from build123d import *

# Parameters (mm, degrees)
SKETCH1_R           = 12.7
SKETCH1_R_2         = 1.65
BOSS_EXTRUDE1_DEPTH = 12.7
SKETCH2_R           = 1.65
CUT_EXTRUDE1_DEPTH  = 12.7
SKETCH3_R           = 2.77495
CUT_EXTRUDE3_DEPTH  = 1.99898
SKETCH7_R           = 1.65
BOSS_EXTRUDE2_DEPTH = 10.70102
SKETCH8_R           = 1.65
BOSS_EXTRUDE3_DEPTH = 10.70102
SKETCH9_R           = 1.65
BOSS_EXTRUDE4_DEPTH = 10.70102
SKETCH10_R          = 1.65
BOSS_EXTRUDE5_DEPTH = 10.70102
SKETCH12_R          = 1.25
CUT_EXTRUDE4_DEPTH  = 12.7
SKETCH11_R          = 1.25
CUT_EXTRUDE5_DEPTH  = 12.7


with BuildPart() as part:
    # Sketch1 → Boss-Extrude1 (new body)
    with BuildSketch(Plane(origin=(0, 0, 0), x_dir=(1, 0, 0), z_dir=(0, 1, 0))):
        with BuildLine():
            Line((21.686311219, 59.206008809), (23.227161891, 57.665158137))
            ThreePointArc((23.227161891, 57.665158137), (23.323849078, 57.508955756), (23.357596674, 57.328376976))
            Line((23.357596674, 57.328376976), (23.357596674, 26.344510207))
            ThreePointArc((23.357596674, 26.344510207), (23.323849078, 26.163931427), (23.227161891, 26.007729046))
            Line((23.227161891, 26.007729046), (21.686311219, 24.466878374))
            ThreePointArc((21.686311219, 24.466878374), (21.530108838, 24.370191187), (21.349530059, 24.336443591))
            Line((21.349530059, 24.336443591), (-9.634336711, 24.336443591))
            ThreePointArc((-9.634336711, 24.336443591), (-9.814915491, 24.370191187), (-9.971117871, 24.466878374))
            Line((-9.971117871, 24.466878374), (-11.511968543, 26.007729046))
            ThreePointArc((-11.511968543, 26.007729046), (-11.60865573, 26.163931427), (-11.642403326, 26.344510207))
            Line((-11.642403326, 26.344510207), (-11.642403326, 57.328376976))
            ThreePointArc((-11.642403326, 57.328376976), (-11.60865573, 57.508955756), (-11.511968543, 57.665158137))
            Line((-11.511968543, 57.665158137), (-9.971117871, 59.206008809))
            ThreePointArc((-9.971117871, 59.206008809), (-9.814915491, 59.302695995), (-9.634336711, 59.336443591))
            Line((-9.634336711, 59.336443591), (21.349530059, 59.336443591))
            ThreePointArc((21.349530059, 59.336443591), (21.530108838, 59.302695995), (21.686311219, 59.206008809))
        make_face()
        with Locations(Location((5.857596674, 41.836443591, 0), (0, 0, 90))):
            Circle(SKETCH1_R, mode=Mode.SUBTRACT)
        with Locations(Location((18.857596674, 54.836443591, 0), (0, 0, 90))):
            Circle(SKETCH1_R_2, mode=Mode.SUBTRACT)
        with Locations(Location((18.857596674, 28.836443591, 0), (0, 0, 90))):
            Circle(SKETCH1_R_2, mode=Mode.SUBTRACT)
        with Locations(Location((-7.142403326, 54.836443591, 0), (0, 0, 90))):
            Circle(SKETCH1_R_2, mode=Mode.SUBTRACT)
        with Locations(Location((-7.142403326, 28.836443591, 0), (0, 0, 90))):
            Circle(SKETCH1_R_2, mode=Mode.SUBTRACT)
    extrude(amount=BOSS_EXTRUDE1_DEPTH)

    # Sketch2 → Cut-Extrude1 (cut)
    with BuildSketch(Plane.XY.offset(-24.336443591)):
        with Locations((-1.888370018, 6.35)):
            Circle(SKETCH2_R)
        with Locations((13.603563366, 6.35)):
            Circle(SKETCH2_R)
        with Locations((5.857596674, 6.35)):
            Circle(SKETCH2_R)
    extrude(amount=-CUT_EXTRUDE1_DEPTH, mode=Mode.SUBTRACT)

    # Sketch3 → Cut-Extrude3 (cut)
    with BuildSketch(Plane(origin=(0, 12.7, 0), x_dir=(1, 0, 0), z_dir=(0, 1, 0))):
        with Locations(Location((-7.142403326, 54.836443591, 0), (0, 0, 270))):
            Circle(SKETCH3_R)
        with Locations(Location((18.857596674, 54.836443591, 0), (0, 0, 270))):
            Circle(SKETCH3_R)
        with Locations(Location((-7.142403326, 28.836443591, 0), (0, 0, 270))):
            Circle(SKETCH3_R)
        with Locations(Location((18.857596674, 28.836443591, 0), (0, 0, 270))):
            Circle(SKETCH3_R)
    extrude(amount=-CUT_EXTRUDE3_DEPTH, mode=Mode.SUBTRACT)

    # Sketch7 → Boss-Extrude2 (add, through all)
    with BuildSketch(Plane(origin=(0, 10.70102, 0), x_dir=(1, 0, 0), z_dir=(0, 1, 0))):
        with Locations((-7.142403326, 28.836443591)):
            Circle(SKETCH7_R)
    extrude(amount=-BOSS_EXTRUDE2_DEPTH)

    # Sketch8 → Boss-Extrude3 (add, through all)
    with BuildSketch(Plane(origin=(0, 10.70102, 0), x_dir=(1, 0, 0), z_dir=(0, 1, 0))):
        with Locations((-7.142403326, 54.836443591)):
            Circle(SKETCH8_R)
    extrude(amount=-BOSS_EXTRUDE3_DEPTH)

    # Sketch9 → Boss-Extrude4 (add, through all)
    with BuildSketch(Plane(origin=(0, 10.70102, 0), x_dir=(1, 0, 0), z_dir=(0, 1, 0))):
        with Locations((18.857596674, 54.836443591)):
            Circle(SKETCH9_R)
    extrude(amount=-BOSS_EXTRUDE4_DEPTH)

    # Sketch10 → Boss-Extrude5 (add, through all)
    with BuildSketch(Plane(origin=(0, 10.70102, 0), x_dir=(1, 0, 0), z_dir=(0, 1, 0))):
        with Locations((18.857596674, 28.836443591)):
            Circle(SKETCH10_R)
    extrude(amount=-BOSS_EXTRUDE5_DEPTH)

    # Sketch12 → Cut-Extrude4 (cut)
    with BuildSketch(Plane(origin=(0, 10.70102, 0), x_dir=(1, 0, 0), z_dir=(0, 1, 0))):
        with Locations(Location((18.857596674, 54.836443591, 0), (0, 0, 270))):
            Circle(SKETCH12_R)
        with Locations(Location((-7.142403326, 28.836443591, 0), (0, 0, 270))):
            Circle(SKETCH12_R)
        with Locations(Location((18.857596674, 28.836443591, 0), (0, 0, 270))):
            Circle(SKETCH12_R)
    extrude(amount=-CUT_EXTRUDE4_DEPTH, mode=Mode.SUBTRACT)

    # Sketch11 → Cut-Extrude5 (cut)
    with BuildSketch(Plane(origin=(0, 10.70102, 0), x_dir=(1, 0, 0), z_dir=(0, 1, 0))):
        with Locations(Location((-7.142403326, 54.836443591, 0), (0, 0, 270))):
            Circle(SKETCH11_R)
    extrude(amount=-CUT_EXTRUDE5_DEPTH, mode=Mode.SUBTRACT)


solid = part.part
Read the model definition and answer for the solid it produces. Units are mm, in the model's axes. A direction names the side the tool comes from. Coordinates: 2 decimals unless noted, no trailing zeros. Loops run counter-clockwise (first coordinate to the right, second up) from the corner with the lowest first, then second, coordinate; pieces in that order, holes last.
Q1. The mould has two halves that part along X. Classify faces 1 (the face through (22.446, 6.261, -58.446)), 2 (the face through (-3.537, 6.423, -27.757)), 3 (the face through (-11.642, 6, -42)): +X half, -X half, draft (parallel to the pull), parting line (faces both ways), or undercut.
Q2. The part is cut by section C-C on z = -49.5. Write down the section's boundary in (x, y).
Q3. Which of the six approach directions +Z, -Z, +X, -X, +Y, -Y give full straight-line access (tool end or side, diameter ignored) to faces 4 (the face through (2.04, 6.26, -53.95)), 5 (the face through (20, 10.701, -54)), 6 (the face through (4.548, 5.346, -26.756))?
Q4. Consider probe 1 along X at (y, z) = (11.5, -29); probe 2 along Z at (x, y) = (19.5, 4); probe 3 along Z at (x, y) = (15, 5). Determine where each line is inside the solid, lowest interval first.
Q5. The part is cut by section A-A on y = 6.35. Give the number of separate pieces and of enclosed holes in the cut face, and give its area (3 significant figures).
Q6. Each of these flat-tipped pins is pushed along its axis until it touches: pin 1 Ø3 at (x, z) = (-7.14, -28.84) entering from -Y; pin 2 Ø3 at (x, z) = (18.86, -28.84) entering from +Y. Where does it stop, or does it pass through?
Q7. The part is cut by section B-B on x = 7. Write down the section's boundary in (y, z).
Q8. The part is cut by section D-D on y = 4. Write down the section's boundary in (x, z).
Results below:
1. face 1: +X half
1. face 2: undercut
1. face 3: -X half
2. outline: (-11.64, 0) - (-4.27, 0) - (-4.27, 12.7) - (-11.64, 12.7) - close; (15.98, 0) - (23.36, 0) - (23.36, 12.7) - (15.98, 12.7) - close
3. face 4: +Y, -Y
3. face 5: +Y
3. face 6: +Z
4. probe 1: x = -11.64 to -9.91, -4.37 to 16.09, 21.63 to 23.36
4. probe 2: z = -59.34 to -55.91, -53.76 to -29.91, -27.76 to -24.34
4. probe 3: z = -59.34 to -50.65, -33.02 to -24.34
5. separate pieces: 3
5. enclosed holes: 4
5. area: 627 mm2
6. pin 1: stops at y = 0
6. pin 2: stops at y = 10.7
7. outline: (0, -59.34) - (12.7, -59.34) - (12.7, -54.48) - (0, -54.48) - close; (0, -29.19) - (5.16, -29.19) - (5.16, -24.34) - (0, -24.34) - close; (7.54, -29.19) - (12.7, -29.19) - (12.7, -24.34) - (7.54, -24.34) - close
8. outline: (-11.64, -57.33) arc R0.5 ccw to (-11.51, -57.67) - (-9.97, -59.21) arc R0.5 ccw to (-9.63, -59.34) - (21.35, -59.34) arc R0.5 ccw to (21.69, -59.21) - (23.23, -57.67) arc R0.5 ccw to (23.36, -57.33) - (23.36, -26.34) arc R0.5 ccw to (23.23, -26.01) - (21.69, -24.47) arc R0.5 ccw to (21.35, -24.34) - (-9.63, -24.34) arc R0.5 ccw to (-9.97, -24.47) - (-11.51, -26.01) arc R0.5 ccw to (-11.64, -26.34) - close; hole circle Ø2.5 at (-7.14, -54.84); hole circle Ø2.5 at (-7.14, -28.84); hole circle Ø25.4 at (5.86, -41.84); hole circle Ø2.5 at (18.86, -54.84); hole circle Ø2.5 at (18.86, -28.84)
